Part model, mm, in its own coordinate system. A direction names the side the tool comes from. Coordinates: 2 decimals unless noted, no trailing zeros. Order: outer loops, then holes, each group sorted by start corner. A loop starts at its lowest first (then second) coordinate and runs counter-clockwise, first axis right, second up.
1) Tool access for faces 4 (the flat face through (678, -401.196, 3)), 5 (the flat face through (621, -415.296, 3)): list every direction of +Z, -Z, +X, -X, +Y, -Y with a clear straight run to the whole face (end or side of a thin tool).
2) Cut at B-B (x = 650). List the corners of the cut face in (y, z), and give its area (3 significant figures).
3) Pin check, flat tips, straight feed: pin 1 Ø1.8 at (y, z) = (-406.5, 4) entering from +X; pin 2 Ø1.5 at (y, z) = (-435.5, 3.5) entering from +X; pin 3 Ø1.8 at (x, z) = (604.5, 4) entering from +Y; pin 4 Ø1.9 at (x, y) = (657.53, -432.28) entering from -Z. Stop position of each tip, or through.
4) Mould opens along X. For faces 1 (the cylindrical face through (681.821, -440.282, 2.958)), 2 (the flat face through (567.751, -408, 3)), 3 (the flat face through (621, -428, 0)) say: +X half, -X half, draft (parallel to the pull), parting line (faces both ways), or undercut.
5) Wall check: L1, parallel to Y at x = 625, z = 3.25; L2, parallel to X at y = -431, z = 4; L3, parallel to X at y = -403.5, z = 2.25. Give the ranges that are in metal, low to high.
6) Cut at A-A (y = -414). List the corners of the cut face in (x, z).
7) Cut at C-C (y = -439.5). List the corners of the cut face in (x, z), and give its area (3 significant figures).
8) Cut at D-D (z = 5). Give the number of separate pieces and of enclosed holes in the cut face, and give its area (3 significant figures).
```python
from build123d import *

# Parameters (mm, degrees)
DODANIE_WYCI_GNI_CIE1_DEPTH = 6
SZKIC5_R                    = 1.55
WYTNIJ_WYCI_GNI_CIE4_DEPTH  = 6
WYTNIJ_WYCI_GNI_CIE3_DEPTH  = 10
WYTNIJ_WYCI_GNI_CIE5_DEPTH  = 6


with BuildPart() as part:
    # Szkic1 → Dodanie-wyciągnięcie1 (new body)
    with BuildSketch(Plane.XY):
        with BuildLine():
            Line((559.30310538, -401.196233577), (679.169206808, -401.196233577))
            add(Edge.make_bspline(
                [(687.47449185, -407.105172623), (687.460895427, -406.945083018), (687.399523084, -406.440112421), (687.106391165, -405.247306424), (686.199030087, -403.66784482), (684.728358654, -402.453584158), (683.321816891, -401.804200876), (682.065878557, -401.467025134), (680.947934354, -401.299453727), (680.131685922, -401.236634896), (679.578376244, -401.210432629), (679.339173948, -401.201842063), (679.210839256, -401.19761192), (679.187499025, -401.196838314), (679.169206808, -401.196233577)],
                knots=[0.021401383, 0.021401383, 0.021401383, 0.021401383, 0.051544166, 0.115122874, 0.24228029, 0.369437707, 0.496595123, 0.62375254, 0.750909956, 0.878067373, 0.941646081, 0.990181611, 0.996198883, 1.005224789, 1.005224789, 1.005224789, 1.005224789], degree=3))
            Line((687.47449185, -407.105172623), (687.524116, -407.588097358))
            Line((687.524116, -407.588097358), (687.524116, -419.296173359))
            Line((687.524116, -419.296173359), (687.524116, -426.296170097))
            ThreePointArc((687.524116, -426.296170097), (681.666251932, -440.438306105), (667.524116585, -446.296171768))
            Line((667.524116585, -446.296171768), (572.829457094, -446.296179681))
            ThreePointArc((572.829457094, -446.296179681), (558.687321683, -440.438316102), (552.829456509, -426.296181352))
            Line((552.829456509, -426.296181352), (552.829456509, -407.696232795))
            Line((552.829456509, -407.696232795), (552.829456509, -407.111536822))
            ThreePointArc((552.829456509, -407.111536822), (554.918503283, -402.897768775), (559.30310538, -401.196233577))
        make_face()
    extrude(amount=DODANIE_WYCI_GNI_CIE1_DEPTH)

    # Szkic5 → Wytnij-wyciągnięcie4 (cut)
    with BuildSketch(Plane.XY.offset(6)):
        with Locations((582.829456509, -432.296173588)):
            Circle(SZKIC5_R)
        with Locations((657.534304884, -432.275447832)):
            Circle(SZKIC5_R)
    extrude(amount=-WYTNIJ_WYCI_GNI_CIE4_DEPTH, mode=Mode.SUBTRACT)

    # Szkic4 → Wytnij-wyciągnięcie3 (cut)
    with BuildSketch(Plane.XY.offset(6)):
        with BuildLine():
            Line((598.90310538, -405.068549386), (592.90310538, -405.068549386))
            ThreePointArc((592.90310538, -405.068549386), (590.428231646, -406.093675652), (589.40310538, -408.568549386))
            Line((589.40310538, -408.568549386), (589.40310538, -409.168549386))
            ThreePointArc((589.40310538, -409.168549386), (590.428231646, -411.64342312), (592.90310538, -412.668549386))
            Line((592.90310538, -412.668549386), (598.90310538, -412.668549386))
            ThreePointArc((598.90310538, -412.668549386), (601.377979114, -411.64342312), (602.40310538, -409.168549386))
            Line((602.40310538, -409.168549386), (602.40310538, -408.568549386))
            ThreePointArc((602.40310538, -408.568549386), (601.377979114, -406.093675652), (598.90310538, -405.068549386))
        make_face()
    extrude(amount=-WYTNIJ_WYCI_GNI_CIE3_DEPTH, mode=Mode.SUBTRACT)

    # Szkic7 → Wytnij-wyciągnięcie5 (cut)
    with BuildSketch(Plane.XY.offset(6)):
        with BuildLine():
            Line((668.604116, -415.296173181), (571.751345179, -415.296173181))
            ThreePointArc((571.751345179, -415.296173181), (568.922918055, -414.124600305), (567.751345179, -411.296173181))
            Line((567.751345179, -411.296173181), (567.751345179, -405.196233577))
            ThreePointArc((567.751345179, -405.196233577), (566.579772304, -402.367806452), (563.751345179, -401.196233577))
            Line((563.751345179, -401.196233577), (676.593615823, -401.192611842))
            ThreePointArc((676.593615823, -401.192611842), (673.771978935, -402.367885748), (672.604116, -405.19259806))
            Line((672.604116, -405.19259806), (672.604116, -411.296173181))
            ThreePointArc((672.604116, -411.296173181), (671.432543125, -414.124600305), (668.604116, -415.296173181))
        make_face()
    extrude(amount=-WYTNIJ_WYCI_GNI_CIE5_DEPTH, mode=Mode.SUBTRACT)


solid = part.part
```
Geometry check:
1. face 4: +Z, -Z, +X, -X, +Y
1. face 5: +Z, -Z, +Y
2. outline: (-446.3, 0) - (-415.3, 0) - (-415.3, 6) - (-446.3, 6) - close
2. area: 186 mm2
3. pin 1: stops at x = 687.5
3. pin 2: stops at x = 685.65
3. pin 3: stops at y = -415.3
3. pin 4: passes through
4. face 1: +X half
4. face 2: undercut
4. face 3: draft
5. L1: y = -446.3 to -415.3
5. L2: x = 553.39 to 581.98, 583.68 to 656.65, 658.42 to 686.96
5. L3: x = 554.34 to 567.37, 672.98 to 685.89
6. outline: (552.83, 0) - (568.8, 0) - (568.8, 6) - (552.83, 6) - close; (671.55, 0) - (687.52, 0) - (687.52, 6) - (671.55, 6) - close
7. outline: (557.81, 0) - (682.55, 0) - (682.55, 6) - (557.81, 6) - close
7. area: 748 mm2
8. separate pieces: 1
8. enclosed holes: 2
8. area: 4,390 mm2
